Verification items for the finished model (mm, model axes). Face numbers are marked on the shaded views. Round coordinates to 2 decimals unless told otherwise and drop trailing zeros. Write each loop counter-clockwise with the first axis right and the second up, starting at its lowest first coordinate (ties: lowest second). Pieces come first, ordered by that corner, then holes. Notation, with made-up numbers: (21, 11.25) - (34, 11.25) arc R25 ccw to (34, 43.25) - close; hole circle Ø10 at (-28, 32). An arc over 180 degrees is marked (long way). Answer as a JSON object with one key per item and string values. Group by question number.
1) Go/stop test with flat-tipped pins: pin 1 Ø2 at (x, y) = (-28, 33) entering from +Z; pin 2 Ø2 at (x, y) = (-5, 43) entering from -Z; pin 3 Ø12 at (x, z) = (20.5, 27) entering from +Y. Record where each tip stops, or that it passes through.
2) Section check D-D (y = 43.5). Enter the section's corners in (x, z), then the cut area to 3 significant figures.
3) Thickness scan on line 1 (X direction, y = 8, z = 0); line 2 (X direction, y = 26.5, z = 0.5); line 3 (X direction, y = 16.5, z = 34.5). Record the ranges inside material, lowest first.
4) Section check A-A (x = 0). Enter the section's corners in (y, z).
5) Section check B-B (z = 0). Enter the section's corners in (x, y), then the cut area to 3 significant figures.
6) Section check C-C (y = 14.5). Enter the section's corners in (x, z).
7) Mould release check, pull along Z, two halves, no side actions. Record for the marked faces 1, 2 and 3: +Z half, -Z half, draft (parallel to the pull), parting line (faces both ways), or undercut.
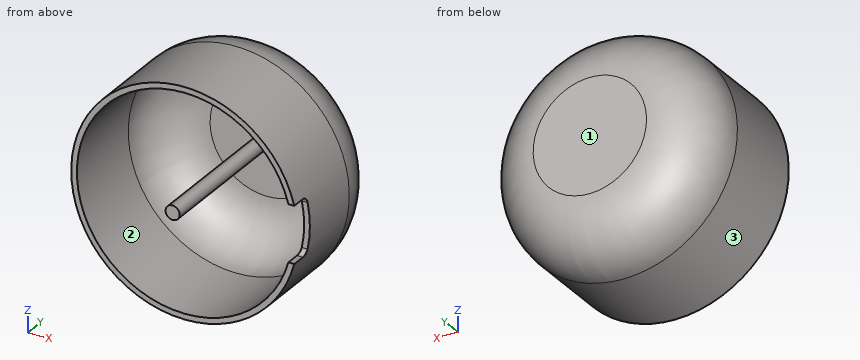
```python
from build123d import *

# Parameters (mm, degrees)
SHELL1_T            = -2
SKETCH2_R           = 2.5
BOSS_EXTRUDE1_DEPTH = 55
CUT_EXTRUDE2_DEPTH  = 50


with BuildPart() as part:
    # Sketch1 → Revolve1 (revolve)
    with BuildSketch(Plane(origin=(0, 0, 0), x_dir=(0, 0, -1), z_dir=(1, 0, 0))):
        with BuildLine():
            Line((0, 0), (0, 50))
            Line((0, 50), (20, 50))
            ThreePointArc((20, 50), (34.142135624, 44.142135624), (40, 30))
            Line((40, 30), (40, 0))
            Line((40, 0), (0, 0))
        make_face()
    revolve(axis=Axis((0, 0, 0), (0, 1, 0)))

    # Shell1
    shell1_openings = [part.faces().sort_by_distance(p)[0] for p in [
        (0, 0, 0),
    ]]
    offset(amount=SHELL1_T, openings=shell1_openings, kind=Kind.INTERSECTION)

    # Sketch2 → Boss-Extrude1 (add)
    with BuildSketch(Plane.XZ.offset(-48)):
        with Locations(Location((0, 0, 0), (0, 0, 90))):
            Circle(SKETCH2_R)
    extrude(amount=BOSS_EXTRUDE1_DEPTH)

    # Sketch3 → Cut-Extrude2 (cut)
    with BuildSketch(Plane(origin=(6, 0, 0), x_dir=(0, 0, -1), z_dir=(1, 0, 0))):
        with BuildLine():
            Line((-10, 0), (10, 0))
            Line((10, 0), (10, 5))
            ThreePointArc((10, 5), (9.414213562, 6.414213562), (8, 7))
            Line((8, 7), (-8, 7))
            ThreePointArc((-8, 7), (-9.414213562, 6.414213562), (-10, 5))
            Line((-10, 5), (-10, 0))
        make_face()
    extrude(amount=CUT_EXTRUDE2_DEPTH, mode=Mode.SUBTRACT)


solid = part.part
```
Returned:
{
 "1": {"pin 1": "z = 29.23", "pin 2": "z = -35.66", "pin 3": "y = 48.37"},
 "2": {"outline": "circle Ø69.51 at (0, 0); circle Ø5 at (0, 0); hole circle Ø63.81 at (0, 0)", "area": "617 mm2"},
 "3": {"line 1": "-40 to -38, -2.5 to 2.5, 38 to 40", "line 2": "-40 to -38, -2.45 to 2.45, 38 to 40", "line 3": "-20.24 to -15.93, 15.93 to 20.24"},
 "4": {"outline": "(-7, -2.5) - (48, -2.5) - (48, -20) arc R18 cw to (30, -38) - (0, -38) - (0, -40) - (30, -40) arc R20 ccw to (50, -20) - (50, 20) arc R20 ccw to (30, 40) - (0, 40) - (0, 38) - (30, 38) arc R18 cw to (48, 20) - (48, 2.5) - (-7, 2.5) - close"},
 "5": {"outline": "(-40, 0) - (-38, 0) - (-38, 30) arc R18 cw to (-20, 48) - (-2.5, 48) - (-2.5, -7) - (2.5, -7) - (2.5, 48) - (20, 48) arc R18 cw to (38, 30) - (38, 7) - (40, 7) - (40, 30) arc R20 ccw to (20, 50) - (-20, 50) arc R20 ccw to (-40, 30) - close", "area": "580 mm2"},
 "6": {"outline": "circle Ø80 at (0, 0); circle Ø5 at (0, 0); hole circle Ø76 at (0, 0)"},
 "7": {"face 1": "draft", "face 2": "undercut", "face 3": "parting line"}
}
